Read the model definition and answer for the solid it produces. Units are mm, in the model's axes. A direction names the side the tool comes from. Round coordinates to 2 decimals unless told otherwise and drop trailing zeros. Order: outer loops, then holes, each group sorted by start corner. A loop starts at its lowest first (then second) coordinate and runs counter-clockwise, first axis right, second up. Notation, with made-up numbers: (52, -21) - (94, -21) arc R33 cw to (94, 13) - close; hole circle Ø8 at (6, -21). An arc over 180 degrees is marked (long way). Put each result on its own line as item: value. Start each with the question number.
Q1. Section C-C on z = -0.75 is taken. Give the vertices of the cut face in (x, y).
Q2. For a pull along X with two mould halves and no side action, classify faces 1 (the face through (2.5, 6, 0)), 2 (the face through (0, 6, 0)), 3 (the face through (1, 6, -2.625)) as pulls with the +X half, pulls with the -X half, needs draft (parallel to the pull), parting line crosses it, or undercut.
Q3. Which of the six approach directions +Z, -Z, +X, -X, +Y, -Y give full straight-line access (tool end or side, diameter ignored) to faces 4 (the face through (-3.747, -1.374, 0.433)), 5 (the face through (1.232, -2.624, 0.058))?
Q4. Find the intervals of material crossed by line 1 along X through (y, z) = (5, -0.3); line 2 along Y through (x, z) = (-1.25, -0.05); line 3 along Z through (x, y) = (-0.5, 1.25), in increasing order. Write a range as from..to.
Q5. Section D-D on z = -1.7 is taken. Give the vertices of the cut face in (x, y), then the cut area to 3 significant figures.
Q6. Section A-A on y = -0.75 is taken. Give the vertices of the cut face in (x, z), then the cut area to 3 significant figures.
Q7. Each of these flat-tipped pins is pushed along its axis until it touches: pin 1 Ø4 at (x, y) = (-3.5, 4.5) entering from +Z; pin 2 Ø1 at (x, y) = (-2.5, 1.5) entering from +Z; pin 3 Ø1.5 at (y, z) = (2, 1.5) entering from -X. Where does it stop, or does it pass through?
Q8. Section B-B on x = -1.5 is taken. Give the vertices of the cut face in (y, z), then the cut area to 3 significant figures.
from build123d import *

# Parameters (mm, degrees)
F1_DEPTH = 2.5
F2_R     = 1.44
F3_DEPTH = 7.6


with BuildPart() as f1:
    # F0 (on Right) → F1 (new body)
    with BuildSketch(Plane.YZ):
        with BuildLine():
            ThreePointArc((0, -2.625), (1.856155, -1.856155), (2.625, 0))
            ThreePointArc((2.625, 0), (1.856155, 1.856155), (0, 2.625))
            ThreePointArc((0, 2.625), (-2.625, 0), (0, -2.625))
        make_face()
        with BuildLine():
            ThreePointArc((0, 2.625), (1.856155, 1.856155), (2.625, 0))
            ThreePointArc((2.625, 0), (1.856155, -1.856155), (0, -2.625))
            Line((0, -2.625), (13.125, -2.625))
            Line((13.125, -2.625), (14.745, 2.625))
            Line((14.745, 2.625), (0, 2.625))
        make_face()
    extrude(amount=F1_DEPTH)

    # F2 (on face) → F3 (join)
    with BuildSketch(Plane(origin=(0, 0, 0), x_dir=(0, -1, 0), z_dir=(-1, 0, 0))):
        Circle(F2_R)
    extrude(amount=F3_DEPTH)


solid = f1.part
Findings:
1. outline: (-7.6, -1.23) - (0, -1.23) - (0, -2.52) - (2.5, -2.52) - (2.5, 13.7) - (0, 13.7) - (0, 1.23) - (-7.6, 1.23) - close
2. face 1: pulls with the +X half
2. face 2: pulls with the -X half
2. face 3: needs draft
3. face 4: -X
3. face 5: +X, -X, -Y
4. line 1: 0..2.5
4. line 2: -1.44..1.44
4. line 3: -0.71..0.71
5. outline: (0, -2) - (2.5, -2) - (2.5, 13.41) - (0, 13.41) - close
5. area: 38.5 mm2
6. outline: (-7.6, -1.23) - (0, -1.23) - (0, -2.52) - (2.5, -2.52) - (2.5, 2.52) - (0, 2.52) - (0, 1.23) - (-7.6, 1.23) - close
6. area: 31.3 mm2
7. pin 1: through
7. pin 2: z = 1.04
7. pin 3: x = 0
8. outline: circle Ø2.88 at (0, 0)
8. area: 6.51 mm2
